The listing builds one solid part. Answer for the finished solid, in the listing's coordinates (mm). Face numbers are marked on the shaded views. A direction names the side the tool comes from. Coordinates: 2 decimals unless noted, no trailing zeros. Write each loop counter-clockwise with the first axis right and the second up, starting at its lowest first coordinate (ties: lowest second). Pieces come first, ordered by that corner, then holes.
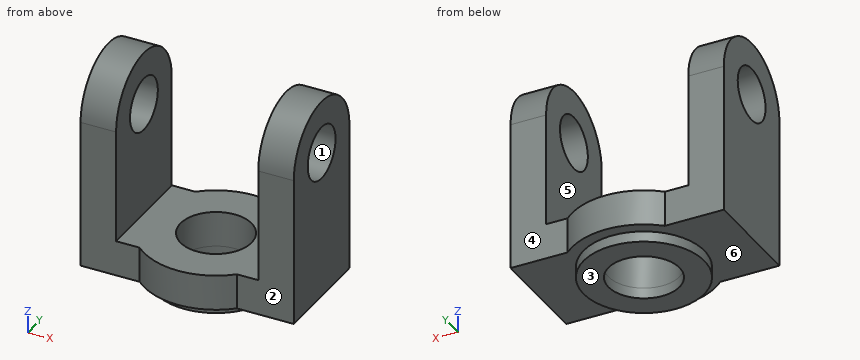
from build123d import *

# Parameters (mm, degrees)
F0_W           = 60
F0_H           = 30
F1_DEPTH       = 10
F2_R           = 10
F3_DEPTH       = 10
F4_R           = 10
F5_DEPTH       = 10
F5_DEPTH_BACK  = 17.75
F6_R           = 17
F7_DEPTH       = 3
F8_R           = 10
F9_DEPTH       = 25
F10_W          = 10
F10_H          = 32
F11_DEPTH      = 5.0168695525
F11_DEPTH_BACK = 24.9831304475
F13_START      = 19.7067023069
F13_DEPTH      = 10
F14_START      = -20.2932976931
F14_DEPTH      = 10
F15_R          = 7.5
F16_DEPTH      = 44.75
F16_DEPTH_BACK = 50.75


with BuildPart() as f1:
    # F0 (on Top) → F1 (new body)
    with BuildSketch(Plane.XY):
        with Locations((-0.2932976931, 9.9831304475)):
            Rectangle(F0_W, F0_H)
    extrude(amount=F1_DEPTH)

    # F2 (on Top) → F3 (join)
    with BuildSketch(Plane.XY):
        with BuildLine():
            ThreePointArc((13.6898891806, 24.9831304475), (0, 30.2910861737), (-13.6898891806, 24.9831304475))
            Line((-13.6898891806, 24.9831304475), (13.6898891806, 24.9831304475))
        make_face()
        with BuildLine():
            Line((13.6898891806, 24.9831304475), (-13.6898891806, 24.9831304475))
            ThreePointArc((-13.6898891806, 24.9831304475), (-18.2871818958, 18.8144408875), (-20.2599732919, 11.3783178851))
            ThreePointArc((-20.2599732919, 11.3783178851), (-18.8506984819, 2.4290433073), (-13.6898891806, -5.0168695525))
            Line((-13.6898891806, -5.0168695525), (13.6898891806, -5.0168695525))
            ThreePointArc((13.6898891806, -5.0168695525), (18.6883022663, 2.0357771662), (20.300634623, 10.52838239))
            ThreePointArc((20.300634623, 10.52838239), (18.4681851426, 18.4293842511), (13.6898891806, 24.9831304475))
        make_face()
        with Locations((0, 9.9831304475)):
            Circle(F2_R, mode=Mode.SUBTRACT)
        with BuildLine():
            Line((13.6898891806, -5.0168695525), (-13.6898891806, -5.0168695525))
            ThreePointArc((-13.6898891806, -5.0168695525), (0, -10.3248252786), (13.6898891806, -5.0168695525))
        make_face()
    extrude(amount=F3_DEPTH)

    # F4 (on Top) → F5 (cut, two sides)
    with BuildSketch(Plane.XY) as f5_sk:
        with Locations((0, 9.9831304475)):
            Circle(F4_R)
    extrude(amount=F5_DEPTH, mode=Mode.SUBTRACT)
    extrude(f5_sk.sketch, amount=-F5_DEPTH_BACK, mode=Mode.SUBTRACT)

    # F6 (on Top) → F7 (join)
    with BuildSketch(Plane.XY):
        with Locations((0, 9.9831304475)):
            Circle(F6_R)
    extrude(amount=-F7_DEPTH)

    # F8 (on Top) → F9 (cut)
    with BuildSketch(Plane.XY):
        with Locations((0, 9.9831304475)):
            Circle(F8_R)
    extrude(amount=-F9_DEPTH, mode=Mode.SUBTRACT)

    # F10 (on Front) → F11 (join, two sides)
    with BuildSketch(Plane.XZ) as f11_sk:
        with Locations((-25.2932976931, 26)):
            Rectangle(F10_W, F10_H)
        with Locations((24.7067023069, 26)):
            Rectangle(F10_W, F10_H)
    extrude(amount=F11_DEPTH)
    extrude(f11_sk.sketch, amount=-F11_DEPTH_BACK)

    # F12 (on Right) → F13 (join)
    with BuildSketch(Plane.YZ.offset(F13_START)):
        with BuildLine():
            ThreePointArc((24.9831304473, 42), (9.9831304473, 57), (-5.0168695527, 42))
            Line((-5.0168695527, 42), (24.9831304473, 42))
        make_face()
    extrude(amount=F13_DEPTH)

    # F12 (on Right) → F14 (join)
    with BuildSketch(Plane.YZ.offset(F14_START)):
        with BuildLine():
            ThreePointArc((24.9831304473, 42), (9.9831304473, 57), (-5.0168695527, 42))
            Line((-5.0168695527, 42), (24.9831304473, 42))
        make_face()
    extrude(amount=-F14_DEPTH)

    # F15 (on Right) → F16 (cut, two sides)
    with BuildSketch(Plane.YZ) as f16_sk:
        with Locations((9.9831304473, 42)):
            Circle(F15_R)
    extrude(amount=-F16_DEPTH, mode=Mode.SUBTRACT)
    extrude(f16_sk.sketch, amount=F16_DEPTH_BACK, mode=Mode.SUBTRACT)


solid = f1.part
Q1. Find the intervals of material crossed by probe 1 along X at (y, z) = (6, 12); probe 2 along Y at (x, z) = (0, -1.1); probe 3 along Y at (x, z) = (26.5, 42), in increasing order.
Answers below:
probe 1: x = -30.29 to -20.29, 19.71 to 29.71
probe 2: y = -7.02 to -0.02, 19.98 to 26.98
probe 3: y = -5.02 to 2.48, 17.48 to 24.98
Q2. The part is cut by section C-C, the plane x = -22. Write down the section's boundary in (y, z), then the cut area to 3 significant figures.
Answers below:
outline: (-5.02, 0) - (24.98, 0) - (24.98, 42) arc R15 ccw to (-5.02, 42) - close; hole circle Ø15 at (9.98, 42)
area: 1,440 mm2
Q3. Determine the mould class of the marked faces 1, 2 and 3 for opening direction Z: released by +Z, released by -Z, zero draft, split by the parting line, or undercut.
Answers below:
face 1: undercut
face 2: zero draft
face 3: released by -Z
Q4. The part is cut by section B-B, the plane y = 22.5. Write down the section's boundary in (x, z).
Answers below:
outline: (-30.29, 0) - (-11.5, 0) - (-11.5, -3) - (11.5, -3) - (11.5, 0) - (29.71, 0) - (29.71, 50.27) - (19.71, 50.27) - (19.71, 10) - (-20.29, 10) - (-20.29, 50.27) - (-30.29, 50.27) - close
Q5. Which of the six approach directions +Z, -Z, +X, -X, +Y, -Y give full straight-line access (tool end or side, diameter ignored) to the marked faces 4, 5 and 6?
Answers below:
face 4: +Z, -Z, +X, +Y
face 5: +Z, +Y, -Y
face 6: -Z
Q6. Given pin 1 (19.5 mm diameter, centred on y = 9.98, z = 42, fed in from +X); pin 2 (2 mm diameter, centred on x = -21.5, z = 47.5, fed in from -Y); pin 3 (13.5 mm diameter, centred on y = 9.98, z = 42, fed in from +X) (3 decimals); pin 4 (17.5 mm diameter, centred on x = 20, z = 23.5, fed in from -Y), each flat-ended and moving along its own axis, determine where each tip first touches the part or whether it passes through.
Answers below:
pin 1: stops at x = 29.71
pin 2: stops at y = -4.33
pin 3: passes through
pin 4: stops at y = -5.02
Q7. The part is cut by section D-D, the plane y = 5. Write down the section's boundary in (x, z).
Answers below:
outline: (-30.29, 0) - (-16.25, 0) - (-16.25, -3) - (-8.67, -3) - (-8.67, 10) - (-20.29, 10) - (-20.29, 36.39) - (-30.29, 36.39) - close; (-30.29, 47.61) - (-20.29, 47.61) - (-20.29, 56.15) - (-30.29, 56.15) - close; (8.67, -3) - (16.25, -3) - (16.25, 0) - (29.71, 0) - (29.71, 36.39) - (19.71, 36.39) - (19.71, 10) - (8.67, 10) - close; (19.71, 47.61) - (29.71, 47.61) - (29.71, 56.15) - (19.71, 56.15) - close
Q8. The part is cut by section A-A, the plane x = 0. Write down the section's boundary in (y, z).
Answers below:
outline: (-10.32, 0) - (-7.02, 0) - (-7.02, -3) - (-0.02, -3) - (-0.02, 10) - (-10.32, 10) - close; (19.98, -3) - (26.98, -3) - (26.98, 0) - (30.29, 0) - (30.29, 10) - (19.98, 10) - close
